Autodesk Fusion 360 part; units mm, degrees
ref_plane "工作平面1" through (0, 0, 0) normal (0, 0, 1) x (1, 0, 0)
sketch "草图1" plane through (0, 0, 0) normal (0, 0, 1) x (1, 0, 0)
  line L0 (-26, -22) -> (26, -22)
  line L1 (26, -22) -> (28, -20)
  line L2 (28, -20) -> (28, 20)
  line L3 (28, 20) -> (26, 22)
  line L4 (26, 22) -> (-26, 22)
  line L5 (-26, 22) -> (-28, 20)
  line L6 (-28, 20) -> (-28, -20)
  line L7 (-28, -20) -> (-26, -22)
extrude "56 x 44 x 7 platform" add sketch "草图1" along normal blind 12
ref_plane "工作平面2" through (0, 0, 12) normal (0, 0, 1) x (1, 0, 0)
sketch "草图2" plane through (0, 0, 12) normal (0, 0, 1) x (1, 0, 0)
  line L0 (-28, -22) -> (-20.49, -22)
  line L1 (-20.49, -22) -> (-20.49, 22)
  line L2 (-20.49, 22) -> (-28, 22)
  line L3 (-28, 22) -> (-28, -22)
ref_plane "工作平面3" through (0, 0, 17.2) normal (0, 0, 1) x (1, 0, 0)
sketch "草图3" plane through (0, 0, 17.2) normal (0, 0, 1) x (1, 0, 0)
  line L0 (-28, -22) -> (-16.33, -22)
  line L1 (-16.33, -22) -> (-16.33, 22)
  line L2 (-16.33, 22) -> (-28, 22)
  line L3 (-28, 22) -> (-28, -22)
loft "Dovetail retaining rail 0.8 to 1 -1" add profiles "草图2", "草图3" section 1 section 2
ref_plane "工作平面4" through (0, 0, 11.7) normal (0, 0, 1) x (1, 0, 0)
sketch "草图4" plane through (0, 0, 11.7) normal (0, 0, 1) x (1, 0, 0)
  line L0 (-23.4, -22) -> (-22.5, -22)
  line L1 (-22.5, -22) -> (-22.5, 13)
  line L2 (-22.5, 13) -> (-23.4, 13)
  line L3 (-23.4, 13) -> (-23.4, -22)
extrude "0.9 mm longitudinal flexure slot -1" cut sketch "草图4" along normal blind 5.8
ref_plane "工作平面5" through (0, 0, 11.7) normal (0, 0, 1) x (1, 0, 0)
sketch "草图5" plane through (0, 0, 11.7) normal (0, 0, 1) x (1, 0, 0)
  line L0 (-22.5, -22) -> (-15, -22)
  line L1 (-15, -22) -> (-15, 13)
  line L2 (-15, 13) -> (-22.5, 13)
  line L3 (-22.5, 13) -> (-22.5, -22)
extrude "0.8 mm flexure underside relief -1" cut sketch "草图5" along normal blind 0.8
ref_plane "工作平面6" through (0, 0, 12.6) normal (0, 0, 1) x (1, 0, 0)
sketch "草图6" plane through (0, 0, 12.6) normal (0, 0, 1) x (1, 0, 0)
  line L0 (-20.21, -6) -> (-20.21, 11)
  line L1 (-20.21, 11) -> (-19.66, 11)
  line L2 (-19.66, 11) -> (-19.66, 2)
  line L3 (-19.66, 2) -> (-20.11, -6)
  line L4 (-20.11, -6) -> (-20.21, -6)
ref_plane "工作平面7" through (0, 0, 16.8) normal (0, 0, 1) x (1, 0, 0)
sketch "草图7" plane through (0, 0, 16.8) normal (0, 0, 1) x (1, 0, 0)
  line L0 (-16.85, -6) -> (-16.85, 11)
  line L1 (-16.85, 11) -> (-16.3, 11)
  line L2 (-16.3, 11) -> (-16.3, 2)
  line L3 (-16.3, 2) -> (-16.75, -6)
  line L4 (-16.75, -6) -> (-16.85, -6)
loft "Tapered friction contact rib -1" add profiles "草图6", "草图7" section 1 section 2
ref_plane "工作平面8" through (0, 0, 12) normal (0, 0, 1) x (1, 0, 0)
sketch "草图8" plane through (0, 0, 12) normal (0, 0, 1) x (1, 0, 0)
  line L0 (20.49, -22) -> (28, -22)
  line L1 (28, -22) -> (28, 22)
  line L2 (28, 22) -> (20.49, 22)
  line L3 (20.49, 22) -> (20.49, -22)
ref_plane "工作平面9" through (0, 0, 17.2) normal (0, 0, 1) x (1, 0, 0)
sketch "草图9" plane through (0, 0, 17.2) normal (0, 0, 1) x (1, 0, 0)
  line L0 (16.33, -22) -> (28, -22)
  line L1 (28, -22) -> (28, 22)
  line L2 (28, 22) -> (16.33, 22)
  line L3 (16.33, 22) -> (16.33, -22)
loft "Dovetail retaining rail 0.8 to 1 1" add profiles "草图8", "草图9" section 1 section 2
ref_plane "工作平面10" through (0, 0, 11.7) normal (0, 0, 1) x (1, 0, 0)
sketch "草图10" plane through (0, 0, 11.7) normal (0, 0, 1) x (1, 0, 0)
  line L0 (22.5, -22) -> (23.4, -22)
  line L1 (23.4, -22) -> (23.4, 13)
  line L2 (23.4, 13) -> (22.5, 13)
  line L3 (22.5, 13) -> (22.5, -22)
extrude "0.9 mm longitudinal flexure slot 1" cut sketch "草图10" along normal blind 5.8
ref_plane "工作平面11" through (0, 0, 11.7) normal (0, 0, 1) x (1, 0, 0)
sketch "草图11" plane through (0, 0, 11.7) normal (0, 0, 1) x (1, 0, 0)
  line L0 (15, -22) -> (22.5, -22)
  line L1 (22.5, -22) -> (22.5, 13)
  line L2 (22.5, 13) -> (15, 13)
  line L3 (15, 13) -> (15, -22)
extrude "0.8 mm flexure underside relief 1" cut sketch "草图11" along normal blind 0.8
ref_plane "工作平面12" through (0, 0, 12.6) normal (0, 0, 1) x (1, 0, 0)
sketch "草图12" plane through (0, 0, 12.6) normal (0, 0, 1) x (1, 0, 0)
  line L0 (20.21, -6) -> (20.21, 11)
  line L1 (20.21, 11) -> (19.66, 11)
  line L2 (19.66, 11) -> (19.66, 2)
  line L3 (19.66, 2) -> (20.11, -6)
  line L4 (20.11, -6) -> (20.21, -6)
ref_plane "工作平面13" through (0, 0, 16.8) normal (0, 0, 1) x (1, 0, 0)
sketch "草图13" plane through (0, 0, 16.8) normal (0, 0, 1) x (1, 0, 0)
  line L0 (16.85, -6) -> (16.85, 11)
  line L1 (16.85, 11) -> (16.3, 11)
  line L2 (16.3, 11) -> (16.3, 2)
  line L3 (16.3, 2) -> (16.75, -6)
  line L4 (16.75, -6) -> (16.85, -6)
loft "Tapered friction contact rib 1" add profiles "草图12", "草图13" section 1 section 2
ref_plane "工作平面14" through (0, 0, 12) normal (0, 0, 1) x (1, 0, 0)
sketch "草图14" plane through (0, 0, 12) normal (0, 0, 1) x (1, 0, 0)
  line L0 (-16.5, 19.4) -> (16.5, 19.4)
  line L1 (16.5, 19.4) -> (16.5, 22)
  line L2 (16.5, 22) -> (-16.5, 22)
  line L3 (-16.5, 22) -> (-16.5, 19.4)
extrude "Closed insertion end stop" add sketch "草图14" along normal blind 5.2
ref_plane "工作平面15" through (0, 0, 0) normal (0, 0, 1) x (1, 0, 0)
sketch "草图15" plane through (0, 0, 0) normal (0, 0, 1) x (1, 0, 0)
  circle A0 centre (0, 0) radius 7.5
extrude "15 mm screw and driver access" cut sketch "草图15" along normal blind 12
move_body "Align camera long edge with gimbal arm - 90 degrees" bodies 1 to x (0, 1, 0) y (-1, 0, 0) z (0, 0, 1) at (0, 0, 0)
ref_plane "工作平面16" through (0, 0, 0) normal (0, 0, 1) x (1, 0, 0)
sketch "草图16" plane through (0, 0, 0) normal (0, 0, 1) x (1, 0, 0)
  line L0 (7.8, 5.95) -> (11.4, 5.95)
  line L1 (11.4, 5.95) -> (11.4, 21.05)
  line L2 (11.4, 21.05) -> (7.8, 21.05)
  line L3 (7.8, 21.05) -> (7.8, 5.95)
extrude "Clear original raised tab and root fillet" cut sketch "草图16" along normal blind 11.9
ref_plane "工作平面17" through (0, 0, -2.1) normal (0, 0, 1) x (1, 0, 0)
sketch "草图17" plane through (0, 0, -2.1) normal (0, 0, 1) x (1, 0, 0)
  line L0 (-8.5, -20) -> (-6.3, -20)
  line L1 (-6.3, -20) -> (-6.3, 20)
  line L2 (-6.3, 20) -> (-8.5, 20)
  line L3 (-8.5, 20) -> (-8.5, -20)
extrude "Arm lateral locating shoulder" add sketch "草图17" along normal blind 2.1
ref_plane "工作平面18" through (0, 0, -2.1) normal (0, 0, 1) x (1, 0, 0)
sketch "草图18" plane through (0, 0, -2.1) normal (0, 0, 1) x (1, 0, 0)
  line L0 (8.3, -20) -> (10.5, -20)
  line L1 (10.5, -20) -> (10.5, 20)
  line L2 (10.5, 20) -> (8.3, 20)
  line L3 (8.3, 20) -> (8.3, -20)
extrude "Arm lateral locating shoulder (1)" add sketch "草图18" along normal blind 2.1
ref_plane "工作平面19" through (0, 0, -5.5) normal (0, 0, 1) x (1, 0, 0)
sketch "草图19" plane through (0, 0, -5.5) normal (0, 0, 1) x (1, 0, 0)
  circle A0 centre (0, -24) radius 1.1
extrude "Reinforced 2.2 x 5.5 mm heat stake pin at arm y -4" add sketch "草图19" along normal blind 5.5
ref_plane "工作平面20" through (0, 0, -5.5) normal (0, 0, 1) x (1, 0, 0)
sketch "草图20" plane through (0, 0, -5.5) normal (0, 0, 1) x (1, 0, 0)
  circle A0 centre (0, -16) radius 1.1
extrude "Reinforced 2.2 x 5.5 mm heat stake pin at arm y 4" add sketch "草图20" along normal blind 5.5
ref_plane "工作平面21" through (0, 0, -5.5) normal (0, 0, 1) x (1, 0, 0)
sketch "草图21" plane through (0, 0, -5.5) normal (0, 0, 1) x (1, 0, 0)
  circle A0 centre (0, -10) radius 1.1
extrude "Reinforced 2.2 x 5.5 mm heat stake pin at arm y 10" add sketch "草图21" along normal blind 5.5
ref_plane "工作平面22" through (0, 0, -5.5) normal (0, 0, 1) x (1, 0, 0)
sketch "草图22" plane through (0, 0, -5.5) normal (0, 0, 1) x (1, 0, 0)
  circle A0 centre (0, 12) radius 1.1
extrude "Reinforced 2.2 x 5.5 mm heat stake pin at arm y 32" add sketch "草图22" along normal blind 5.5
ref_plane "工作平面23" through (0, 0, 0) normal (0, 0, 1) x (1, 0, 0)
sketch "草图23" plane through (0, 0, 0) normal (0, 0, 1) x (1, 0, 0)
  line L0 (5, -52.15) -> (8.7, -52.15)
  line L1 (8.7, -52.15) -> (8.7, -27.5)
  line L2 (8.7, -27.5) -> (5, -27.5)
  line L3 (5, -27.5) -> (5, -52.15)
extrude "Ear for original 3.2 mm side hole at arm y -28.15" add sketch "草图23" along normal blind 7.2
ref_plane "工作平面24" through (0, 0, 0) normal (0, 0, 1) x (1, 0, 0)
sketch "草图24" plane through (0, 0, 0) normal (0, 0, 1) x (1, 0, 0)
  line L0 (7.8, -52.15) -> (8.9, -52.15)
  line L1 (8.9, -52.15) -> (8.9, -27.5)
  line L2 (8.9, -27.5) -> (7.8, -27.5)
  line L3 (7.8, -27.5) -> (7.8, -52.15)
extrude "Ear relief around original arm root radius" cut sketch "草图24" along normal blind 1.3
ref_plane "工作平面25" through (4.9, 0, 0) normal (1, 0, 0) x (0, 1, 0)
sketch "草图25" plane through (4.9, 0, 0) normal (1, 0, 0) x (0, 0, -1)
  circle A0 centre (-5, -48.15) radius 1.6
extrude "Side rivet full passage clearance" cut sketch "草图25" along normal blind 20
ref_plane "工作平面26" through (2.9, 0, 0) normal (1, 0, 0) x (0, 1, 0)
sketch "草图26" plane through (2.9, 0, 0) normal (1, 0, 0) x (0, 0, -1)
  circle A0 centre (-5, -48.15) radius 2.9
extrude "Side rivet flange counterbore" cut sketch "草图26" along normal blind 2.2
ref_plane "工作平面27" through (0, 0, 0) normal (0, 0, 1) x (1, 0, 0)
sketch "草图27" plane through (0, 0, 0) normal (0, 0, 1) x (1, 0, 0)
  line L0 (5, 12.85) -> (8.7, 12.85)
  line L1 (8.7, 12.85) -> (8.7, 20.85)
  line L2 (8.7, 20.85) -> (5, 20.85)
  line L3 (5, 20.85) -> (5, 12.85)
extrude "Ear for original 3.2 mm side hole at arm y 36.85" add sketch "草图27" along normal blind 7.2
ref_plane "工作平面28" through (0, 0, 0) normal (0, 0, 1) x (1, 0, 0)
sketch "草图28" plane through (0, 0, 0) normal (0, 0, 1) x (1, 0, 0)
  line L0 (7.8, 12.85) -> (8.9, 12.85)
  line L1 (8.9, 12.85) -> (8.9, 20.85)
  line L2 (8.9, 20.85) -> (7.8, 20.85)
  line L3 (7.8, 20.85) -> (7.8, 12.85)
extrude "Ear relief around original arm root radius (1)" cut sketch "草图28" along normal blind 1.3
ref_plane "工作平面29" through (4.9, 0, 0) normal (1, 0, 0) x (0, 1, 0)
sketch "草图29" plane through (4.9, 0, 0) normal (1, 0, 0) x (0, 0, -1)
  circle A0 centre (-5, 16.85) radius 1.6
extrude "Side rivet full passage clearance (1)" cut sketch "草图29" along normal blind 20
ref_plane "工作平面30" through (2.9, 0, 0) normal (1, 0, 0) x (0, 1, 0)
sketch "草图30" plane through (2.9, 0, 0) normal (1, 0, 0) x (0, 0, -1)
  circle A0 centre (-5, 16.85) radius 2.9
extrude "Side rivet flange counterbore (1)" cut sketch "草图30" along normal blind 2.2
move_body "Move outward toward free end 20.0 mm" bodies 1 to x (1, 0, 0) y (0, 1, 0) z (0, 0, 1) at (0, 20, 0)
ref_plane "工作平面31" through (0, 0, -2.11) normal (0, 0, 1) x (1, 0, 0)
sketch "草图31" plane through (0, 0, -2.11) normal (0, 0, 1) x (1, 0, 0)
  line L0 (8.29, 25.95) -> (10.51, 25.95)
  line L1 (10.51, 25.95) -> (10.51, 40.05)
  line L2 (10.51, 40.05) -> (8.29, 40.05)
  line L3 (8.29, 40.05) -> (8.29, 25.95)
extrude "Trim locating shoulder before raised side ear root" cut sketch "草图31" along normal blind 2.11
Work out the finished part from the listing and answer in its coordinate system (mm). A direction names the side the tool comes from. Coordinates: 2 decimals unless noted, no trailing zeros. Write each loop counter-clockwise with the first axis right and the second up, starting at its lowest first coordinate (ties: lowest second). Pieces come first, ordered by that corner, then holes.
1. The part is cut by section A-A, the plane x = 6. Write down the section's boundary in (y, z), and give its area (3 significant figures).
Results list:
outline: (-32.15, 0) - (15.5, 0) - (15.5, 12) - (5, 12) - (5, 11.7) - (-3.4, 11.7) - (-3.4, 17.2) - (-8, 17.2) - (-8, 7.2) - (-32.15, 7.2) - close; (-2.5, 12.5) - (-0.09, 12.5) - (3.67, 17.2) - (-2.5, 17.2) - close; (24.5, 0) - (48, 0) - (48, 17.2) - (43.4, 17.2) - (43.4, 11.7) - (35, 11.7) - (35, 12) - (24.5, 12) - close; (36.33, 17.2) - (40.09, 12.5) - (42.5, 12.5) - (42.5, 17.2) - close; hole circle Ø3.2 at (-28.15, 5); hole circle Ø3.2 at (36.85, 5)
area: 805 mm2
2. Consider line 1 along Y through (x, z) = (-8.5, 15); line 2 along Z through (x, y) = (7.95, 36.85); line 3 along Z through (x, y) = (7.5, 36.85). Determine where each line is inside the solid, lowest interval first.
Results list:
line 1: y = -8 to -3.4, -2.5 to 2.26, 37.74 to 42.5, 43.4 to 48
line 2: z = 1.3 to 3.4, 6.6 to 7.2, 16.55 to 17.2
line 3: z = 0 to 3.4, 6.6 to 11.7, 16.55 to 17.2
3. For faces 5 (the flat face through (4.58, 37.92, 15.21)), 6 (the cylindrical face through (0.33, 12.507, 5.916)), 7 (the cylindrical face through (6.87, 38.27, 4.26)), determine the directions among +Z, -Z, +X, -X, +Y, -Y from which every point of the face is accessible in a straight line to the end or side of a thin tool.
Results list:
face 5: none
face 6: +Z
face 7: +X
4. The part is cut by section C-C, the plane x = 15.5. Write down the section's boundary in (y, z).
Results list:
outline: (-8, 0) - (48, 0) - (48, 17.2) - (43.4, 17.2) - (43.4, 11.7) - (35, 11.7) - (35, 12) - (5, 12) - (5, 11.7) - (-3.4, 11.7) - (-3.4, 17.2) - (-8, 17.2) - close; (-2.5, 12.5) - (-0.09, 12.5) - (3.67, 17.2) - (-2.5, 17.2) - close; (36.33, 17.2) - (40.09, 12.5) - (42.5, 12.5) - (42.5, 17.2) - close; hole circle Ø3.2 at (36.85, 5)
5. The part is cut by section D-D, the plane z = 14.75. State how many separate pieces and enclosed holes the cut face has, and give its area (3 significant figures).
Results list:
separate pieces: 3
enclosed holes: 0
area: 886 mm2
6. The part is cut by section B-B, the plane y = -28.15. Write down the section's boundary in (x, z), and give its area (3 significant figures).
Results list:
outline: (5, 0) - (7.8, 0) - (7.8, 1.3) - (8.7, 1.3) - (8.7, 3.4) - (5.1, 3.4) - (5.1, 2.1) - (5, 2.1) - close; (5.1, 6.6) - (8.7, 6.6) - (8.7, 7.2) - (5.1, 7.2) - close
area: 13.4 mm2
7. For a pull along X with two mould halves and no side action, classify faces 1 (the flat face through (22, 18, 6)), 2 (the flat face through (8.3, 13, -1)), 3 (the flat face through (-8.5, 20, -1)), 4 (the flat face through (0, 48, 9)) as +X half, -X half, draft (parallel to the pull), parting line (faces both ways), or undercut.
Results list:
face 1: +X half
face 2: undercut
face 3: -X half
face 4: draft
8. Flat-ended cylindrical pins translate along their axes: pin 1 (6 mm diameter, centred on y = -21, z = 4, fed in from -X); pin 2 (0.7 mm diameter, centred on x = -1, y = -1.5, fed in from -Z); pin 3 (1.3 mm diameter, centred on x = -7, y = 21.5, fed in from +Z). Find the tip coordinate at first contact, or state that the pin passes through.
Results list:
pin 1: stops at x = 5
pin 2: stops at z = 0
pin 3: stops at z = 12
